Work out the finished part from the listing and answer in its coordinate system (mm). Face numbers are marked on the shaded views. A direction names the side the tool comes from. Give positions to 0.01 mm unless a question says otherwise; leave off trailing zeros. Loops run counter-clockwise (first coordinate to the right, second up) from the corner with the lowest first, then second, coordinate; pieces in that order, holes last.
```python
from build123d import *

# Parameters (mm, degrees)
F0_W        = 22
F0_H        = 11
F1_DEPTH    = 2
F2_W        = 15
F2_H        = 9
F3_DEPTH    = 6
F4_T        = 1.2
F4_T3_DEPTH = 17.4
F4_T5_DEPTH = 11.4
F6_R        = 1
F7_DEPTH    = 25
F5_R        = 1
F8_DEPTH    = 25


# Not quite as in the source:
# - a shell that OpenCascade refuses in one call is made with other operations: the cavity is built on its own and cut out


with BuildPart() as f1:
    # F0 (on Top) → F1 (new body)
    with BuildSketch(Plane.XY):
        with Locations((10.5796571493, 0.5358164497)):
            Rectangle(F0_W, F0_H)
    extrude(amount=F1_DEPTH)

    # F2 (on Top) → F3 (join)
    with BuildSketch(Plane.XY):
        with Locations((10.2674138546, 0.1021951512)):
            Rectangle(F2_W, F2_H)
    extrude(amount=F3_DEPTH)

    # F4: shell of thickness 1.2, made by hand


with BuildPart() as f4_core1:
    # F4_t2: copy of F1
    add(f1.part)

    # the walls: a layer under each face that stays
    f4_faces = [f4_core1.faces().sort_by_distance(p)[0] for p in [
        (10.5796571493, -4.9641835503, 1),
        (-0.4203428507, 0.5358164497, 1),
        (21.5796571493, 0.5358164497, 1),
        (10.5796571493, 0.5358164497, 0),
        (17.9129904826, -3.130850217, 2),
        (10.5796571493, 6.0358164497, 1),
        (10.2674138546, -4.3978048488, 4),
        (17.7674138546, 0.1021951512, 4),
        (10.2674138546, 4.6021951512, 4),
        (2.7674138546, 0.1021951512, 4),
    ]]
    thicken(f4_faces, amount=-F4_T, mode=Mode.SUBTRACT)

    # F4_s4 → F4_t3 (cut)
    with BuildSketch(Plane.YZ.offset(1.5674138546)):
        Polygon((-4.4098048488, 2.012), (-4.3978048488, 0.8), (-3.1978048488, 0.8), (-3.1978048488, 2), align=None)
        Polygon((4.6141951512, 2.012), (4.6021951512, 0.8), (3.4021951512, 0.8), (3.4021951512, 2), align=None)
    extrude(amount=F4_T3_DEPTH, mode=Mode.SUBTRACT)

    # F4_s6 → F4_t5 (cut)
    with BuildSketch(Plane.XZ.offset(-5.8021951512)):
        Polygon((17.7794138546, 2.012), (17.7674138546, 0.8), (16.5674138546, 0.8), (16.5674138546, 2), align=None)
        Polygon((2.7554138546, 2.012), (2.7674138546, 0.8), (3.9674138546, 0.8), (3.9674138546, 2), align=None)
    extrude(amount=F4_T5_DEPTH, mode=Mode.SUBTRACT)


with BuildPart() as f1_1:
    add(f1.part)

    # what is left inside the walls is the cavity
    f4_cavity = [f4_core1.part.solids().sort_by_distance(p)[0] for p in [
        (10.267414, -0.997805, 1.212),
    ]]
    add(f4_cavity, mode=Mode.SUBTRACT)

    # F6 (on face) → F7 (cut)
    with BuildSketch(Plane.XY.offset(2)):
        with Locations((19.5883829147, 0)):
            Circle(F6_R)
    extrude(amount=-F7_DEPTH, mode=Mode.SUBTRACT)

    # F5 (on face) → F8 (cut)
    with BuildSketch(Plane.XY.offset(2)):
        with Locations((1.0301771374, -0.018063417)):
            Circle(F5_R)
    extrude(amount=-F8_DEPTH, mode=Mode.SUBTRACT)


solid = f1_1.part
```
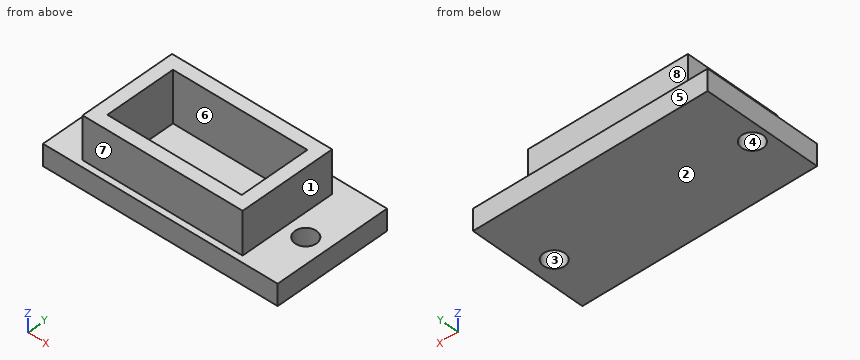
Q1. Consider line 1 along X through (y, z) = (-1, 2.55); line 2 along Y through (x, z) = (16.5, 3.9); line 3 along X through (y, z) = (3, 1.3). Determine where each line is inside the solid, lowest interval first.
Q2. Section A-A on x = 19.75 is taken. Give the vertices of the cut face in (y, z), plus the area to 3 significant figures.
Q3. Determine the mould class of the marked faces 1, 2 and 3 for opening direction X: +X half, -X half, draft (parallel to the pull), parting line (faces both ways), or undercut.
Q4. Section D-D on x = 8.25 is taken. Give the vertices of the cut face in (y, z).
Q5. Given pin 1 (2.5 mm diameter, centred on x = 11.5, z = 3, fed in from +Y); pin 2 (2 mm diameter, centred on x = 6.5, z = 4.5, fed in from +Y); pin 3 (1.2 mm diameter, centred on y = -1, z = 4.5, fed in from +X); pin 4 (1.6 mm diameter, centred on x = 19.59, y = 0, fed in from -Z), each flat-ended and moving along its own axis, determine where each tip first touches the part or whether it passes through.
Q6. Section C-C on z = 2.85 is taken. Give the vertices of the cut face in (x, y), plus the area to 3 significant figures.
Q7. Section B-B on y = 4 is taken. Give the vertices of the cut face in (x, z), plus the area to 3 significant figures.
Q8. Which of the six approach directions +Z, -Z, +X, -X, +Y, -Y give full straight-line access (tool end or side, diameter ignored) to the marked faces 4, 5, 6, 7 and 8?
Check result:
1. line 1: x = 2.77 to 3.97, 16.57 to 17.77
1. line 2: y = -4.4 to -3.2, 3.4 to 4.6
1. line 3: x = -0.42 to 3.97, 16.57 to 21.58
2. outline: (-4.96, 0) - (-0.99, 0) - (-0.99, 2) - (-4.96, 2) - close; (0.99, 0) - (6.04, 0) - (6.04, 2) - (0.99, 2) - close
2. area: 18.1 mm2
3. face 1: +X half
3. face 2: draft
3. face 3: undercut
4. outline: (-4.96, 0) - (6.04, 0) - (6.04, 2) - (4.6, 2) - (4.6, 6) - (3.4, 6) - (3.4, 1.2) - (-3.2, 1.2) - (-3.2, 6) - (-4.4, 6) - (-4.4, 2) - (-4.96, 2) - close
5. pin 1: stops at y = 6.04
5. pin 2: stops at y = 4.6
5. pin 3: stops at x = 17.77
5. pin 4: passes through
6. outline: (2.77, -4.4) - (17.77, -4.4) - (17.77, 4.6) - (2.77, 4.6) - close; hole (3.97, -3.2) - (16.57, -3.2) - (16.57, 3.4) - (3.97, 3.4) - close
6. area: 51.8 mm2
7. outline: (-0.42, 0) - (21.58, 0) - (21.58, 2) - (17.77, 2) - (17.77, 6) - (2.77, 6) - (2.77, 2) - (-0.42, 2) - close
7. area: 104 mm2
8. face 4: +Z, -Z
8. face 5: +Z, -Z, +X, -X, +Y
8. face 6: +Z
8. face 7: +Z, +X, -X, -Y
8. face 8: +Z, +X, -X, +Y
